```python
from build123d import *

# Parameters (mm, degrees)
RESSALTO_EXTRUS_O1_DEPTH = 48
ESBO_O12_R               = 1.5
CORTE_EXTRUS_O10_DEPTH   = 10
ESBO_O13_R               = 1.5
CORTE_EXTRUS_O11_DEPTH   = 10
ESBO_O14_R               = 1.5
CORTE_EXTRUS_O12_DEPTH   = 10
ESBO_O15_R               = 1.5
CORTE_EXTRUS_O13_DEPTH   = 10
CORTE_EXTRUS_O14_DEPTH   = 10
ESBO_O17_R               = 4
ESBO_O17_W               = 2.8
ESBO_O17_H               = 2.8
RESSALTO_EXTRUS_O2_DEPTH = 4
CORTE_EXTRUS_O15_DEPTH   = 10


with BuildPart() as part:
    # Model → Ressalto-extrusão1 (new body)
    with BuildSketch(Plane.XY):
        with BuildLine():
            Line((-0.7, 0), (39, 0))
            Line((39, 0), (39.7, 0))
            Line((39.7, 0), (39.7, -11.380317396))
            Line((39.7, -11.380317396), (50.182424304, -21.8627417))
            Line((50.182424304, -21.8627417), (58.119682605, -29.8))
            Line((58.119682605, -29.8), (81.7, -29.8))
            ThreePointArc((81.7, -29.8), (105.905643752, -13.626305928), (100.226197667, 14.926197667))
            Line((100.226197667, 14.926197667), (65.00338056, 50.149014774))
            Line((65.00338056, 50.149014774), (50.111140335, 50.149014774))
            Line((50.111140335, 50.149014774), (14.181595121, 50.149014774))
            Line((14.181595121, 50.149014774), (-3.2, 32.767419653))
            Line((-3.2, 32.767419653), (-3.2, 5))
            Line((-3.2, 5), (-3.2, 0))
            Line((-3.2, 0), (-0.7, 0))
        make_face()
        with BuildLine():
            Line((-0.7, 2.5), (39, 2.5))
            Line((39, 2.5), (39.7, 2.5))
            Line((39.7, 2.5), (42.2, 2.5))
            Line((42.2, 2.5), (42.2, -10.34478349))
            Line((42.2, -10.34478349), (51.950191257, -20.094974747))
            Line((51.950191257, -20.094974747), (59.15521651, -27.3))
            Line((59.15521651, -27.3), (81.7, -27.3))
            ThreePointArc((81.7, -27.3), (103.595944921, -12.669597347), (98.458430714, 13.158430714))
            Line((98.458430714, 13.158430714), (63.967846654, 47.649014774))
            Line((63.967846654, 47.649014774), (50.111140335, 47.649014774))
            Line((50.111140335, 47.649014774), (15.217129027, 47.649014774))
            Line((15.217129027, 47.649014774), (-0.7, 31.731885747))
            Line((-0.7, 31.731885747), (-0.7, 2.5))
        make_face(mode=Mode.SUBTRACT)
    extrude(amount=RESSALTO_EXTRUS_O1_DEPTH)

    # Esboço12 → Corte-extrusão10 (cut)
    with BuildSketch(Plane(origin=(57.576197667, 57.576197667, 0), x_dir=(0, 0, -1), z_dir=(0.707106781, 0.707106781, 0))):
        with Locations((-44, -20.072657306)):
            Circle(ESBO_O12_R)
        with Locations((-44, -52.072657306)):
            Circle(ESBO_O12_R)
    extrude(amount=-CORTE_EXTRUS_O10_DEPTH, mode=Mode.SUBTRACT)

    # Esboço13 → Corte-extrusão11 (cut)
    with BuildSketch(Plane(origin=(0, 50.149014774, 0), x_dir=(1, 0, 0), z_dir=(0, 1, 0))):
        with Locations((39.59248784, -44)):
            Circle(ESBO_O13_R)
    extrude(amount=-CORTE_EXTRUS_O11_DEPTH, mode=Mode.SUBTRACT)

    # Esboço14 → Corte-extrusão12 (cut)
    with BuildSketch(Plane.ZY.offset(3.2)):
        with Locations((44, 23.701037279)):
            Circle(ESBO_O14_R)
        with Locations((44, 7.740898975)):
            Circle(ESBO_O14_R)
    extrude(amount=-CORTE_EXTRUS_O12_DEPTH, mode=Mode.SUBTRACT)

    # Esboço15 → Corte-extrusão13 (cut)
    with BuildSketch(Plane(origin=(14.159841302, 14.159841302, 0), x_dir=(0, 0, 1), z_dir=(-0.707106781, -0.707106781, 0))):
        with Locations((44, -46.881179593)):
            Circle(ESBO_O15_R)
    extrude(amount=-CORTE_EXTRUS_O13_DEPTH, mode=Mode.SUBTRACT)

    # Esboço16 → Corte-extrusão14 (cut)
    with BuildSketch(Plane.XY.offset(48)):
        Polygon((39.7, 0), (39.7, -7.84478349), (42.2, -10.34478349), (42.2, 2.5), (-0.7, 2.5), (-0.7, 0), align=None)
    extrude(amount=-CORTE_EXTRUS_O14_DEPTH, mode=Mode.SUBTRACT)

    # Esboço17 → Ressalto-extrusão2 (add)
    with BuildSketch(Plane(origin=(0, 0, 0), x_dir=(-1, 0, 0), z_dir=(0, 0, -1))):
        with Locations((-91.568699638, 17.926841447)):
            Circle(ESBO_O17_R)
        with Locations((-91.568699638, 17.926841447)):
            Rectangle(ESBO_O17_W, ESBO_O17_H, mode=Mode.SUBTRACT)
        with Locations((-68.47265349, 41.022887595)):
            Circle(ESBO_O17_R)
        with Locations((-68.47265349, 41.022887595)):
            Rectangle(ESBO_O17_W, ESBO_O17_H, mode=Mode.SUBTRACT)
        with Locations((-39.59248784, 46.149014774)):
            Circle(ESBO_O17_R)
        with Locations((-39.59248784, 46.149014774)):
            Rectangle(ESBO_O17_W, ESBO_O17_H, mode=Mode.SUBTRACT)
        with Locations((-0.8, 24.383709827)):
            Circle(ESBO_O17_R)
        with Locations((-0.8, 24.383709827)):
            Rectangle(ESBO_O17_W, ESBO_O17_H, mode=Mode.SUBTRACT)
        with Locations((-0.8, 8.383709827)):
            Circle(ESBO_O17_R)
        with Locations((-0.8, 8.383709827)):
            Rectangle(ESBO_O17_W, ESBO_O17_H, mode=Mode.SUBTRACT)
        with Locations((-51.388268427, -17.411731573)):
            Circle(ESBO_O17_R)
        with Locations((-51.388268427, -17.411731573)):
            Rectangle(ESBO_O17_W, ESBO_O17_H, mode=Mode.SUBTRACT)
    extrude(amount=-RESSALTO_EXTRUS_O2_DEPTH)

    # Esboço18 → Corte-extrusão15 (cut)
    with BuildSketch(Plane.XY.offset(48)):
        Polygon((-0.7, 31.731885747), (-32.431885747, 0), (-0.7, 0), align=None)
    extrude(amount=-CORTE_EXTRUS_O15_DEPTH, mode=Mode.SUBTRACT)

    # Esboço19 → Corte-Revolução1 (revolve, cut)
    with BuildSketch(Plane.ZY.offset(3.2)):
        with BuildLine():
            Line((19, 0), (29, 0))
            Line((29, 0), (38.25689259, 0))
            Line((38.25689259, 0), (38.25689259, 8))
            Line((38.25689259, 8), (24, 8))
            ThreePointArc((24, 8), (20.464466094, 6.535533906), (19, 3))
            Line((19, 3), (19, 0))
        make_face()
    revolve(axis=Axis((-3.2, 0, 19), (0, 0, 1)), mode=Mode.SUBTRACT)


solid = part.part
```
Here's how the part is built. I have some questions about the finished solid (model axes, mm). A direction names the side the tool comes from. Coordinates: 2 decimals unless noted, no trailing zeros. Order: outer loops, then holes, each group sorted by start corner. A loop starts at its lowest first (then second) coordinate and runs counter-clockwise, first axis right, second up.
1) Imagine slicing it at B-B on z = 44. State how many separate pieces and enclosed holes the cut face has, and give its area (3 significant figures).
2) Will these pins go through, and if not, where does the flat tip stop? pin 1 (23.5 mm diameter, centred on y = 20.5, z = 11, fed in from +X); pin 2 (3 mm diameter, centred on x = 34.5, z = 32, fed in from -Y); pin 3 (2 mm diameter, centred on x = 69, z = 2, fed in from +Y).
3) Imagine slicing it at A-A on x = 23. List the corners of the cut face in (y, z) for me.
4) We'd pull the mould along X, two halves only. Please class faces 5 (the face through (1, 22.984, 2)), 6 (the face through (82.86, 32.29, 23.66)), 7 (the face through (3, 8, 4)), 8 (the face through (40, 1, 0)): +X half, -X half, draft (parallel to the pull), parting line (faces both ways), or undercut.
5) I need wall thicknesses on line 1 (Y direction, x = 39, z = 2); line 2 (Y direction, x = 59.5, z = 40); line 3 (Y direction, x = 35, z = 12.5). Which ranges of each line are inside material? Lowest first, please.
6) Imagine slicing it at D-D on x = 6. List the corners of the cut face in (y, z) for me, and give its area (3 significant figures).
7) Imagine slicing it at C-C on z = 10.5. List the corners of the cut face in (x, y) for me.
8) Which directions (+Z, -Z, +X, -X, +Y, -Y) give clear straight access to the entire face, cutting with the end or side of a thin tool? Please do faces 1 (the face through (40.992, 46, 2)), 2 (the face through (81, 31, 48)), 3 (the face through (40, 44, 4)), 4 (the face through (40.285, 48.917, 45.331)).
Response values:
1. separate pieces: 5
1. enclosed holes: 0
1. area: 553 mm2
2. pin 1: stops at x = 104.81
2. pin 2: stops at y = 0
2. pin 3: stops at y = 47.15
3. outline: (0, 0) - (2.5, 0) - (2.5, 38) - (0, 38) - close; (47.65, 0) - (50.15, 0) - (50.15, 48) - (47.65, 48) - close
4. face 5: undercut
4. face 6: +X half
4. face 7: undercut
4. face 8: draft
5. line 1: y = 0 to 2.5, 42.19 to 44.75, 47.55 to 50.15
5. line 2: y = -29.8 to -27.3, 47.65 to 50.15
5. line 3: y = 0 to 2.5, 47.65 to 50.15
6. outline: (0, 0) - (2.5, 0) - (2.5, 38) - (0, 38) - close; (38.43, 0) - (41.97, 0) - (41.97, 48) - (38.43, 48) - close
6. area: 265 mm2
7. outline: (-3.2, 0) - (39.7, 0) - (39.7, -11.38) - (58.12, -29.8) - (81.7, -29.8) arc R26.2 ccw to (100.23, 14.93) - (65, 50.15) - (14.18, 50.15) - (-3.2, 32.77) - close; hole (-0.7, 2.5) - (42.2, 2.5) - (42.2, -10.34) - (59.16, -27.3) - (81.7, -27.3) arc R23.7 ccw to (98.46, 13.16) - (63.97, 47.65) - (15.22, 47.65) - (-0.7, 31.73) - close
8. face 1: +Z, -Z
8. face 2: +Z, +X, -X, +Y, -Y
8. face 3: +Z
8. face 4: +Y
